Check sheet for the modelled part. Datum: model origin and axes. Units: mm. Face numbers are marked on the shaded views. A direction names the side the tool comes from. Round coordinates to 2 decimals unless told otherwise and drop trailing zeros. Loops run counter-clockwise (first coordinate to the right, second up) from the corner with the lowest first, then second, coordinate; pieces in that order, holes last. Notation, with made-up numbers: (-33.75, 77.25) - (-23.75, 77.25) arc R15 cw to (-23.75, 106.25) - close; hole circle Ø6 at (80, 80.5). An arc over 180 degrees is marked (long way). Put each result on its own line as item: value.
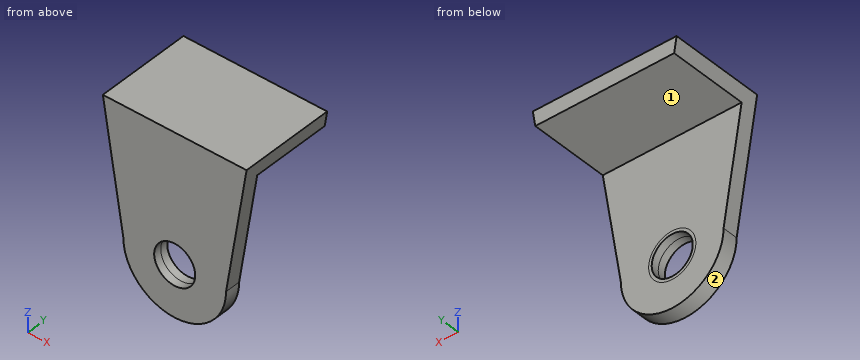
```python
from build123d import *

# Parameters (mm, degrees)
BOSS_EXTRUDE1_DEPTH = 3
SKETCH2_R           = 4
CUT_EXTRUDE1_DEPTH  = 13
BOSS_EXTRUDE2_DEPTH = 15.5
SKETCH6_R           = 4.6
CUT_EXTRUDE4_DEPTH  = 1.5
SKETCH7_R           = 4.6
SKETCH7_R_2         = 4
BOSS_EXTRUDE3_DEPTH = 1.5


with BuildPart() as part:
    # Sketch1 → Boss-Extrude1 (new body)
    with BuildSketch(Plane(origin=(0, 0, 0), x_dir=(1, 0, 0), z_dir=(0, 1, 0))):
        with BuildLine():
            Line((-10, 0), (-14, -25))
            Line((-14, -25), (14, -25))
            Line((14, -25), (10, 0))
            ThreePointArc((10, 0), (0, 10), (-10, 0))
        make_face()
    extrude(amount=BOSS_EXTRUDE1_DEPTH)

    # Sketch2 → Cut-Extrude1 (cut)
    with BuildSketch(Plane(origin=(0, 3, 0), x_dir=(1, 0, 0), z_dir=(0, 1, 0))):
        Circle(SKETCH2_R)
    extrude(amount=-CUT_EXTRUDE1_DEPTH, mode=Mode.SUBTRACT)

    # Sketch5 → Boss-Extrude2 (add)
    with BuildSketch(Plane(origin=(0, 3, 0), x_dir=(1, 0, 0), z_dir=(0, 1, 0))):
        Polygon((-13.52, -22), (13.52, -22), (14, -25), (-14, -25), align=None)
    extrude(amount=BOSS_EXTRUDE2_DEPTH)

    # Sketch6 → Cut-Extrude4 (cut)
    with BuildSketch(Plane(origin=(0, 3, 0), x_dir=(1, 0, 0), z_dir=(0, 1, 0))):
        Circle(SKETCH6_R)
    extrude(amount=-CUT_EXTRUDE4_DEPTH, mode=Mode.SUBTRACT)

    # Sketch7 → Boss-Extrude3 (add)
    with BuildSketch(Plane(origin=(0, 1.5, 0), x_dir=(1, 0, 0), z_dir=(0, 1, 0))):
        Circle(SKETCH7_R)
        Circle(SKETCH7_R_2, mode=Mode.SUBTRACT)
    extrude(amount=BOSS_EXTRUDE3_DEPTH)


solid = part.part
```
Item 1: Thickness scan on line 1 (X direction, y = 1.2, z = 0); line 2 (Z direction, x = 0, y = 2.1); line 3 (Z direction, x = 8.5, y = 17.5). Record the ranges inside material, lowest first. Write a range as from..to.
Filled sheet:
line 1: -10..-4, 4..10
line 2: -10..-4, 4..25
line 3: 22..25
Item 2: Section check B-B on z = 1. Enter the section's corners in (x, y).
Filled sheet:
outline: (-10.16, 0) - (-3.87, 0) - (-3.87, 3) - (-10.16, 3) - close; (3.87, 0) - (10.16, 0) - (10.16, 3) - (3.87, 3) - close
Item 3: Tool access check on the marked faces 1 and 2. Record the directions out of +Z, -Z, +X, -X, +Y, -Y that give a thin tool (end or side, any length) a straight path to the whole face; none if there is none.
Filled sheet:
face 1: -Z, +X, -X, +Y
face 2: -Z, +Y, -Y
Item 4: Section check D-D on y = 6.25. Enter the section's corners in (x, z), then the cut area to 3 significant figures.
Filled sheet:
outline: (-14, 25) - (-13.52, 22) - (13.52, 22) - (14, 25) - close
area: 82.6 mm²
Item 5: Section check C-C on x = -12. Enter the section's corners in (y, z).
Filled sheet:
outline: (0, 12.5) - (3, 12.5) - (3, 22) - (18.5, 22) - (18.5, 25) - (0, 25) - close
Item 6: Section check A-A on x = 0. Enter the section's corners in (y, z), then the cut area to 4 significant figures.
Filled sheet:
outline: (0, -10) - (3, -10) - (3, -4) - (0, -4) - close; (0, 4) - (3, 4) - (3, 22) - (18.5, 22) - (18.5, 25) - (0, 25) - close
area: 127.5 mm²
Item 7: Go/stop test with flat-tipped pins: pin 1 (8 mm diameter, centred on x = -9.5, y = 3, fed in from -Z); pin 2 (1 mm diameter, centred on x = 8.5, z = -1.5, fed in from +Y); pin 3 (5 mm diameter, centred on y = 5, z = 16.5, fed in from -X). Record where each tip stops, or that it passes through.
Filled sheet:
pin 1: z = -8.35
pin 2: y = 3
pin 3: x = -12.88
